Model file for the job. Use its own axes, mm. Face numbers are marked on the shaded views. Coordinates: 2 decimals unless noted, no trailing zeros.
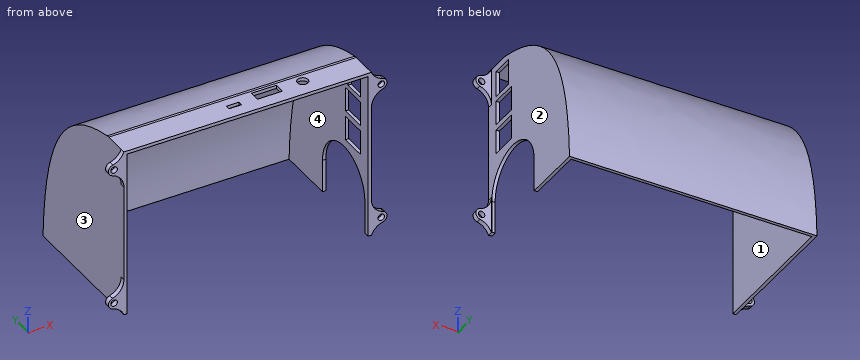
from build123d import *

# Parameters (mm, degrees)
SKETCH2_W           = 151
SKETCH2_H           = 104
BOSS_EXTRUDE1_DEPTH = 2
BOSS_EXTRUDE2_DEPTH = 151
SHELL1_T            = -2
SKETCH4_R           = 3.25
CUT_EXTRUDE1_DEPTH  = 10
SKETCH5_W           = 15
SKETCH5_H           = 16.25
CUT_EXTRUDE2_DEPTH  = 10
FILLET3_R           = 10
CUT_EXTRUDE3_DEPTH  = 10
SKETCH7_R           = 2
BOSS_EXTRUDE3_DEPTH = 3
FILLET4_DEPTH       = 3
FILLET5_R           = 10
SKETCH9_W           = 147
SKETCH9_H           = 102
CUT_EXTRUDE5_DEPTH  = 10


with BuildPart() as part:
    # Sketch2 → Boss-Extrude1 (new body)
    with BuildSketch(Plane(origin=(0, 0, 0), x_dir=(1, 0, 0), z_dir=(0, 1, 0))):
        with Locations((0, -52)):
            Rectangle(SKETCH2_W, SKETCH2_H)
    extrude(amount=BOSS_EXTRUDE1_DEPTH)

    # Sketch3 → Boss-Extrude2 (add)
    with BuildSketch(Plane.ZY.offset(75.5)):
        with BuildLine():
            Line((0, 86), (0, 2))
            Line((0, 2), (104, 2))
            Line((104, 2), (104, 17))
            add(Edge.make_bspline(
                [(0, 86), (63.599399009, 83.650763879), (95.616153821, 65.97970086), (104, 17)],
                knots=[0, 0, 0, 0, 1, 1, 1, 1], degree=3))
        make_face()
    extrude(amount=-BOSS_EXTRUDE2_DEPTH)

    # Shell1
    shell1_openings = [part.faces().sort_by_distance(p)[0] for p in [
        (0, 43, 0),
    ]]
    offset(amount=SHELL1_T, openings=shell1_openings, kind=Kind.INTERSECTION)

    # Sketch4 → Cut-Extrude1 (cut)
    with BuildSketch(Plane.XY.offset(104)):
        with Locations((39.832226511, 10.9)):
            Circle(SKETCH4_R)
        Polygon((-7.059283816, 10.485810058), (-7.059283816, 7.709546788), (-6.933696011, 7.709546788), (0.586748493, 7.709546788), (0.712336299, 7.709546788), (0.712336299, 10.485810058), (0.586748493, 10.485810058), (-0.123473759, 10.485810058), (-6.223473759, 10.485810058), (-6.933696011, 10.485810058), align=None)
        Polygon((12.260960064, 8.05), (14.595960064, 8.05), (25.670959902, 8.05), (25.770960048, 8.05), (25.770960048, 14.466884605), (25.670960048, 14.466884605), (10.670959945, 14.466884605), (10.570959945, 14.466884605), (10.570959945, 8.05), (10.670960001, 8.05), align=None)
    extrude(amount=-CUT_EXTRUDE1_DEPTH, mode=Mode.SUBTRACT)

    # Sketch5 → Cut-Extrude2 (cut)
    with BuildSketch(Plane(origin=(75.5, 0, 0), x_dir=(0, 0, -1), z_dir=(1, 0, 0))):
        Polygon((-99.83530855, 21.4), (-99.83530855, 7.899), (-83.93530855, 7.899), (-83.93530855, 21.4), (-99.53530855, 21.4), align=None)
        Polygon((-65.884309216, 7.95), (-80.884309216, 7.95), (-80.884309216, 21.65), (-80.884309216, 24.2), (-78.334309216, 24.2), (-65.884309216, 24.2), align=None)
        with Locations((-54.984309216, 16.075)):
            Rectangle(SKETCH5_W, SKETCH5_H)
    extrude(amount=-CUT_EXTRUDE2_DEPTH, mode=Mode.SUBTRACT)

    # Fillet3
    fillet3_edges = [part.edges().sort_by_distance(p)[0] for p in [
        (0, 17, 104),
    ]]
    fillet(fillet3_edges, radius=FILLET3_R)

    # Sketch6 → Cut-Extrude3 (cut)
    with BuildSketch(Plane(origin=(75.5, 0, 0), x_dir=(0, 0, -1), z_dir=(1, 0, 0))):
        with BuildLine():
            Line((-20, 48.5), (0, 48.5))
            Line((0, 48.5), (0, 3.504835596))
            Line((0, 3.504835596), (-19.533546963, 3.504835596))
            ThreePointArc((-19.533546963, 3.504835596), (-42.498791069, 25.766760949), (-20, 48.5))
        make_face()
    extrude(amount=-CUT_EXTRUDE3_DEPTH, mode=Mode.SUBTRACT)

    # Sketch7 → Boss-Extrude3 (add)
    # profile 1 of 4: a face of its own
    with BuildSketch(Plane.XZ):
        with BuildLine():
            Line((75.5, 98), (75.5, 91))
            Line((75.5, 91), (81.5, 91))
            ThreePointArc((81.5, 91), (85, 94.5), (81.5, 98))
            Line((81.5, 98), (75.5, 98))
        make_face()
        with Locations(Location((81.5, 94.5, 0), (0, 0, 270))):
            Circle(SKETCH7_R, mode=Mode.SUBTRACT)
    # profile 2 of 4: a face of its own
    with BuildSketch(Plane.XZ):
        with BuildLine():
            Line((-81.5, 91), (-75.5, 91))
            Line((-75.5, 91), (-75.5, 98))
            Line((-75.5, 98), (-81.5, 98))
            ThreePointArc((-81.5, 98), (-85, 94.5), (-81.5, 91))
        make_face()
        with Locations(Location((-81.5, 94.5, 0), (0, 0, 90))):
            Circle(SKETCH7_R, mode=Mode.SUBTRACT)
    # profile 3 of 4: a face of its own
    with BuildSketch(Plane.XZ):
        with BuildLine():
            Line((-75.5, 6), (-75.5, 13))
            Line((-75.5, 13), (-81.5, 13))
            ThreePointArc((-81.5, 13), (-85, 9.5), (-81.5, 6))
            Line((-81.5, 6), (-75.5, 6))
        make_face()
        with Locations(Location((-81.5, 9.5, 0), (0, 0, 270))):
            Circle(SKETCH7_R, mode=Mode.SUBTRACT)
    # profile 4 of 4: a face of its own
    with BuildSketch(Plane.XZ):
        with BuildLine():
            Line((81.5, 13), (75.5, 13))
            Line((75.5, 13), (75.5, 6))
            Line((75.5, 6), (81.5, 6))
            ThreePointArc((81.5, 6), (85, 9.5), (81.5, 13))
        make_face()
        with Locations(Location((81.5, 9.5, 0), (0, 0, 90))):
            Circle(SKETCH7_R, mode=Mode.SUBTRACT)
    extrude(amount=-BOSS_EXTRUDE3_DEPTH)

    # Fillet4: read off the stored shape, not the designer's step
    # Fillet4 outline → Fillet4 (add)
    with BuildSketch(Plane(origin=(0, 0, 0), x_dir=(1, 0, 0), z_dir=(0, 1, 0))):
        with BuildLine():
            ThreePointArc((-81.5, -13), (-82.024439287, -12.960486011), (-82.537037037, -12.842836248))
            ThreePointArc((-82.537037037, -12.842836248), (-77.449235141, -16.462086818), (-75.5, -22.393796958))
            Line((-75.5, -22.393796958), (-75.5, -13))
            Line((-75.5, -13), (-81.5, -13))
        make_face()
        with BuildLine():
            ThreePointArc((-75.5, 0), (-78.189320969, -3.889565288), (-82.365092102, -6.108596801))
            ThreePointArc((-82.365092102, -6.108596801), (-81.935940825, -6.027255322), (-81.5, -6))
            Line((-81.5, -6), (-75.5, -6))
            Line((-75.5, -6), (-75.5, 0))
        make_face()
    extrude(amount=FILLET4_DEPTH)

    # Fillet5
    # the kernel refuses this fillet: 10 mm, written as the material it adds along each edge
    with BuildSketch(Plane(origin=(75.5, 0, 13), x_dir=(0, 0, 1), z_dir=(0, 1, 0)), Plane(origin=(-75.5, 0, 91), x_dir=(0, 0, -1), z_dir=(0, 1, 0))) as fillet5_piece_1:
        with BuildLine():
            CenterArc((9.393796958, 10), FILLET5_R, 197.235285257, 72.764714743)
            Line((-0.157163752, 7.037037037), (-1.112259823, 6.740740741))
            ThreePointArc((-1.112259823, 6.740740741), (-1, 6), (-1, 0))
            Line((-1, 0), (0, -1))
            Line((0, -1), (9.393796958, -1))
            Line((9.393796958, -1), (9.393796958, 0))
        make_face()
    extrude(amount=3)
    with BuildSketch(Plane(origin=(75.5, 0, 6), x_dir=(0, 0, -1), z_dir=(0, 1, 0)), Plane(origin=(-75.5, 0, 98), x_dir=(0, 0, 1), z_dir=(0, 1, 0))) as fillet5_piece_2:
        with BuildLine():
            CenterArc((9.581126623, -9.33678382), FILLET5_R, 110.984333313, 54.705605323)
            Line((-0.108596801, -6.865092102), (-1.077569144, -6.61792293))
            ThreePointArc((-1.077569144, -6.61792293), (-1, -6), (-1, 0))
            Line((-1, 0), (0, 1))
            ThreePointArc((0, 1), (3, 1), (5.641887338, 0.933678382))
            Line((5.641887338, 0.933678382), (6, 0))
        make_face()
    extrude(amount=3)
    with BuildSketch(Plane(origin=(75.5, 0, 91), x_dir=(0, 0, -1), z_dir=(0, 1, 0))) as fillet5_piece_3:
        with BuildLine():
            CenterArc((9.393796958, -10), FILLET5_R, 90, 72.764714743)
            Line((-0.157163752, -7.037037037), (-1.112259823, -6.740740741))
            ThreePointArc((-1.112259823, -6.740740741), (-1, -6), (-1, 0))
            Line((-1, 0), (0, 1))
            Line((0, 1), (9.393796958, 1))
            Line((9.393796958, 1), (9.393796958, 0))
        make_face()
    extrude(amount=3)
    with BuildSketch(Plane(origin=(75.5, 0, 98), x_dir=(0, 0, 1), z_dir=(0, 1, 0))) as fillet5_piece_4:
        with BuildLine():
            CenterArc((9.581126623, 9.33678382), FILLET5_R, 194.310061364, 54.705605323)
            Line((-0.108596801, 6.865092102), (-1.077569144, 6.61792293))
            ThreePointArc((-1.077569144, 6.61792293), (-1, 6), (-1, 0))
            Line((-1, 0), (0, -1))
            ThreePointArc((0, -1), (3, -1), (5.641887338, -0.933678382))
            Line((5.641887338, -0.933678382), (6, 0))
        make_face()
    extrude(amount=3)

    # Sketch9 → Cut-Extrude5 (cut)
    with BuildSketch(Plane(origin=(0, 2, 0), x_dir=(1, 0, 0), z_dir=(0, 1, 0))):
        with Locations((0, -51)):
            Rectangle(SKETCH9_W, SKETCH9_H)
    extrude(amount=-CUT_EXTRUDE5_DEPTH, mode=Mode.SUBTRACT)


solid = part.part
Q1. Drill centre lines: line 1 (X direction, y = 1.9, z = 94.5); line 2 (X direction, y = 57, z = 74); line 3 (Z direction, x = -81, y = 1). Where is each one in solid material? Low to high.
Answers:
line 1: x = -85 to -83.5, -79.5 to -73.5, 73.5 to 79.5, 83.5 to 85
line 2: x = -75.5 to -73.5, 73.5 to 75.5
line 3: z = 5.65 to 7.56, 11.44 to 13.46, 90.54 to 92.56, 96.44 to 98.35
Q2. Flat gauge pins, fed straight in: P1, Ø10.5, axis at x = -81.5, z = 16.5, coming from the +Y side; P2, Ø2, axis at y = 35, z = 68, coming from the +X side; P3, Ø10, axis at x = 30, z = 18.5, coming from the -Y side; P4, Ø3, axis at x = 81.5, z = 9.5, coming from the +Y side. Where does each tip first touch, or does it go through?
Answers:
P1: stops at y = 3
P2: stops at x = 75.5
P3: stops at y = 82.22
P4: passes through
Q3. Mould opens along X. For the marked faces 1, 2, 3 and 4 say: +X half, -X half, draft (parallel to the pull), parting line (faces both ways), or undercut.
Answers:
face 1: undercut
face 2: +X half
face 3: -X half
face 4: undercut
Q4. Slice it at A-A (z = 94.5). Count the separate pieces of the cut face and the enclosed holes in it, and give its area (3 significant figures).
Answers:
separate pieces: 4
enclosed holes: 0
area: 832 mm2
